Part model, mm, in its own coordinate system. A direction names the side the tool comes from. Round coordinates to 2 decimals unless told otherwise and drop trailing zeros. Order: outer loops, then holes, each group sorted by start corner. A loop starts at its lowest first (then second) coordinate and runs counter-clockwise, first axis right, second up. Notation, with made-up numbers: (41, 26.5) - (81, 26.5) arc R16 cw to (81, 35.5) - close; hole circle Ø4 at (57.5, 71.5). An arc over 180 degrees is marked (long way). Answer as a JSON object with one key per item and string values.
Autodesk Fusion 360 part; units mm, degrees
sketch "Sketch3" plane through (0, 0, 0) normal (0, 1, 0) x (1, 0, 0)
  line L0 (40, -40) -> (-40, -40)
  line L1 (-40, -40) -> (-40, 40)
  line L2 (-40, 40) -> (40, 40)
  line L3 (40, 40) -> (40, -40)
  line L4 (40, -40) -> (-40, 40) construction
  line L5 (-40, -40) -> (40, 40) construction
  line L6 (35, 49.9978) -> (35, -35)
  line L7 (35, -35) -> (-35, -35)
  line L8 (-35, -35) -> (-35, 49.9995)
  dimension "d45" = 80
  dimension "d46" = 80
  dimension "d47" = 5
extrude "Extrude10" add sketch "Sketch3" along normal mid plane 25 contours L0 L1 L2 L3 L6 L7 L8
sketch "Sketch9" plane through (40, 0, 0) normal (1, 0, 0) x (0, 1, 0)
  line L0 (-12.5, -40) -> (12.5, -40)
  line L1 (12.5, -40) -> (12.5, 40)
  line L2 (12.5, 40) -> (-12.5, 40)
  line L3 (-12.5, 40) -> (-12.5, -40)
  line L4 (25, -40) -> (-25, -40)
  line L5 (-25, -40) -> (-25, -30)
  line L6 (-25, -30) -> (25, -30)
  line L7 (25, -30) -> (25, -40)
  line L8 (25, -40) -> (-25, -30) construction
  line L9 (-25, -40) -> (25, -30) construction
  line L10 (0, -30.1567) -> (0, 30.1567)
  point P0 (0, -35)
  dimension "d50" = 10
  dimension "d51" = 5
  dimension "d52" = 25
  dimension "d53" = 50
extrude "Extrude11" add sketch "Sketch9" along normal mid plane 10 contours L0 L1 L3 L4 L6 | L3 L4 L5 L6 | L1 L4 L6 L7
sketch "Sketch10" plane through (0, -25, 0) normal (0, -1, 0) x (1, 0, 0)
  line L0 (35, -40) -> (45, -40)
  line L1 (45, -40) -> (45, -30)
  line L2 (45, -30) -> (35, -30)
  line L3 (35, -30) -> (35, -40)
  line L4 (35, -40) -> (45, -30)
  line L5 (45, -40) -> (40, -35)
  circle A0 centre (40, -35) radius 1.6
  dimension "d56" = 3.2
extrude "Extrude12" cut sketch "Sketch10" against normal blind 64 contours L4 A0 | L4 L5 A0 | L4 L5 A0
sketch "Sketch11" plane through (45, 0, 0) normal (1, 0, 0) x (0, 1, 0)
  line L0 (25, -30) -> (-25, -30)
  line L1 (-25, -30) -> (-25, -40)
  line L2 (-25, -40) -> (25, -40)
  line L3 (25, -40) -> (25, -30)
  line L4 (-25, -40) -> (25, -30)
  line L5 (25, -40) -> (-25, -30)
  circle A0 centre (0, -35) radius 1.6
  dimension "d59" = 3.2
extrude "Extrude13" cut sketch "Sketch11" against normal blind 105 contours L4 L5 A0 | L4 L5 A0 | L4 L5 A0 | L4 L5 A0
extrude "Extrude14" add 1 faces at (11.6667, -4.1667, 35) along direction (0, 0, -1) blind 5
sketch "Sketch12" plane through (0, 0, 40) normal (0, 0, 1) x (-1, 0, 0)
  line L0 (-40, 12.5) -> (-40, -12.5)
  line L1 (-40, -12.5) -> (40, -12.5)
  line L2 (40, -12.5) -> (40, 12.5)
  line L3 (40, 12.5) -> (-40, 12.5)
  circle A0 centre (10, -6) radius 2
  circle A1 centre (-10, -6) radius 2
  circle A2 centre (10, 6) radius 2
  circle A3 centre (-10, 6) radius 2
  dimension "d68" = 4
  dimension "d69" = 10
  dimension "d70" = 6
  dimension "d73" = -20
  dimension "d74" = 12
extrude "Extrude15" cut sketch "Sketch12" against normal blind 5.5 contours A0 | A1 | A2 | A3
equation "d48 = ( 25 / 2 ) * 1 mm"
Item 1: Drop flat-ended pins along their axis: P1, Ø2.5, axis at x = 10, y = -6, coming from the +Z side; P2, Ø12, axis at y = -2.5, z = 16.5, coming from the +X side; P3, Ø5, axis at x = -10, y = 6, coming from the +Z side; P4, Ø1.9, axis at y = 0, z = -35, coming from the +X side. Give the stop position or say it passes through.
Taken from the geometry:
{"P1": "z = 34.5", "P2": "x = 40", "P3": "z = 40", "P4": "through"}
Item 2: Cut at C-C (z = 3.5). Write the cut outline in (x, y), plus the area to 3 significant figures.
Taken from the geometry:
{"outline": "(-40, -12.5) - (-35, -12.5) - (-35, 12.5) - (-40, 12.5) - close; (35, -12.5) - (40, -12.5) - (40, 12.5) - (35, 12.5) - close", "area": "250 mm2"}
Item 3: Cut at A-A (z = -35). Write the cut outline in (x, y).
Taken from the geometry:
{"outline": "(-40, -12.5) - (-35, -12.5) - (-35, -1.6) - (-40, -1.6) - close; (-40, 1.6) - (-35, 1.6) - (-35, 12.5) - (-40, 12.5) - close; (35, -25) - (38.4, -25) - (38.4, -1.6) - (35, -1.6) - close; (35, 1.6) - (38.4, 1.6) - (38.4, 25) - (35, 25) - close; (41.6, -25) - (45, -25) - (45, -1.6) - (41.6, -1.6) - close; (41.6, 1.6) - (45, 1.6) - (45, 25) - (41.6, 25) - close"}
Item 4: Probe L1, parallel to X at y = 6, z = 37; L2, parallel to Y at x = -10, z = 38; L3, parallel to X at y = -6.5, z = -35. List the from-to ranges inside material, lowest first. Write a range as from..to.
Taken from the geometry:
{"L1": "-40..-12, -8..8, 12..40", "L2": "-12.5..-8, -4..4, 8..12.5", "L3": "-40..-35, 35..38.4, 41.6..45"}
Item 5: Cut at D-D (x = -10). Write the cut outline in (y, z), plus the area to 3 significant figures.
Taken from the geometry:
{"outline": "(-12.5, 30) - (12.5, 30) - (12.5, 40) - (8, 40) - (8, 34.5) - (4, 34.5) - (4, 40) - (-4, 40) - (-4, 34.5) - (-8, 34.5) - (-8, 40) - (-12.5, 40) - close", "area": "206 mm2"}
Item 6: Cut at B-B (y = 6). Write the cut outline in (x, z).
Taken from the geometry:
{"outline": "(-40, -40) - (-35, -40) - (-35, 30) - (35, 30) - (35, -40) - (45, -40) - (45, -30) - (40, -30) - (40, 40) - (12, 40) - (12, 34.5) - (8, 34.5) - (8, 40) - (-8, 40) - (-8, 34.5) - (-12, 34.5) - (-12, 40) - (-40, 40) - close; hole circle Ø3.2 at (40, -35)"}
Item 7: Tool access for faces 4 (the flat face through (40, 0, -40)), 5 (the cylindrical face through (-10, -8, 37)), 6 (the flat face through (35, 0, -5)), 7 (the flat face through (40, 0, 5)): list every direction of +Z, -Z, +X, -X, +Y, -Y with a clear straight run to the whole face (end or side of a thin tool).
Taken from the geometry:
{"face 4": "-Z, +X, -X, +Y, -Y", "face 5": "+Z", "face 6": "-Z, +Y, -Y", "face 7": "+Z, +X, +Y, -Y"}
Item 8: Two-plate mould, pull along Z, no slides. Class faces 1 (the cylindrical face through (39.792, 12.325, -33.414)), 2 (the flat face through (0, 0, 30)), 3 (the flat face through (45, 0, -33)): pulls with the +Z half, pulls with the -Z half, needs draft (parallel to the pull), parting line crosses it, or undercut.
Taken from the geometry:
{"face 1": "undercut", "face 2": "pulls with the -Z half", "face 3": "needs draft"}
